Drawing for the job (mm, zero at the part's lowest x, y, z). A direction names the side the tool comes from. Round coordinates to 2 decimals unless told otherwise and drop trailing zeros. Order: outer loops, then holes, each group sorted by start corner. A loop starts at its lowest first (then second) coordinate and runs counter-clockwise, first axis right, second up. Notation, with made-up numbers: (85, 75) - (91, 75) arc R22 ccw to (91, 113) - close; hole circle Ø6 at (59.5, 44). An arc over 180 degrees is marked (long way). One line per question, with ' | ' between items. Start each with the question number.
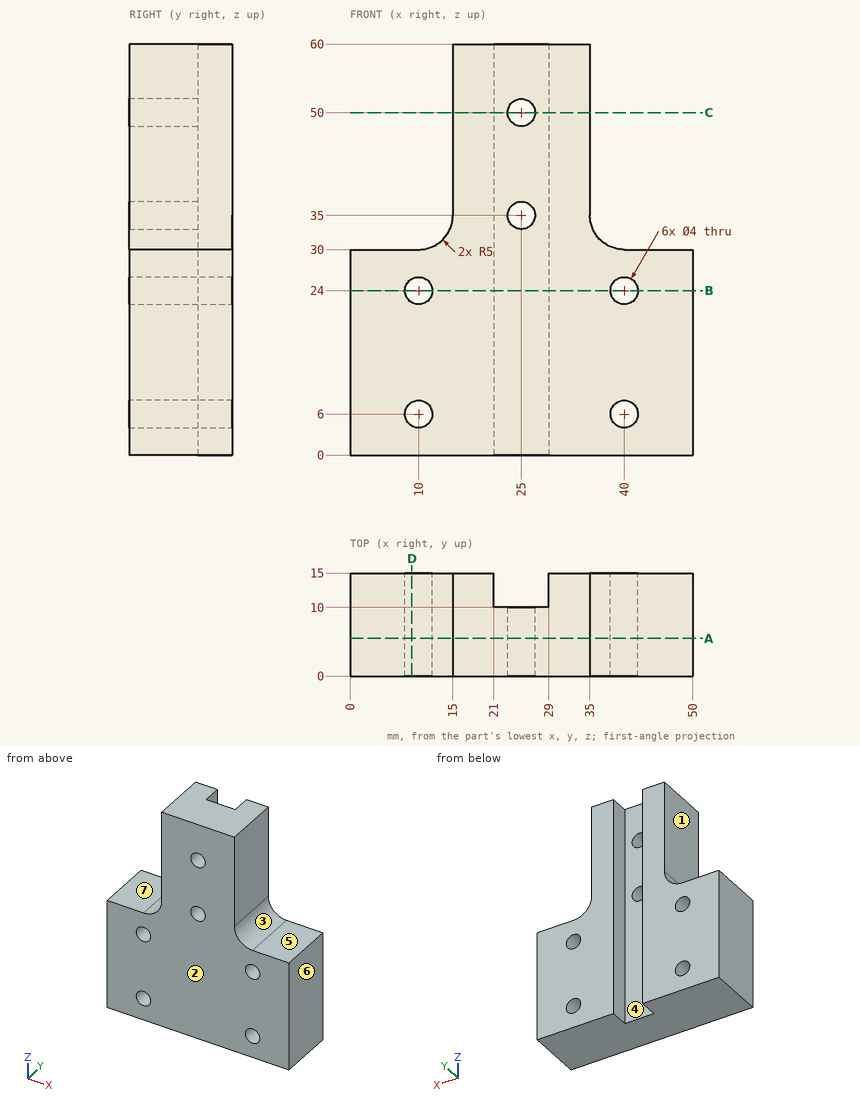
Item 1: Slice it at C-C (z = 50). Write the cut outline in (x, y).
Item 2: Wall check: line 1 along X through (y, z) = (5.75, 24); line 2 along X through (y, z) = (13, 37); line 3 along X through (y, z) = (2, 50). Give the ranges that are in metal, low to high. Write a range as [from, to].
Item 3: Pull direction X, two halves, no side cores. Call the marked faces 1, 2, 3 and 4: released by +X, released by -X, zero draft, split by the parting line, or undercut.
Item 4: 3-axis set-ups, long thin cutter, end or side, ignore diameter. For the marked faces 5, 6 and 7: which of +Z, -Z, +X, -X, +Y, -Y reach the whole face in a straight line?
Item 5: Pin check, flat tips, straight feed: pin 1 (7.5 mm diameter, centred on y = 9.5, z = 45, fed in from +X); pin 2 (5 mm diameter, centred on x = 25, z = 35, fed in from +Y); pin 3 (9 mm diameter, centred on x = 23.5, z = 21.5, fed in from +Y); pin 4 (8 mm diameter, centred on x = 47, y = 6.5, fed in from +Z). Stop position of each tip, or through.
Item 6: Slice it at D-D (x = 9). Write the cut outline in (y, z), plus the area to 3 significant figures.
Item 7: Slice it at B-B (z = 24). Write the cut outline in (x, y).
Item 8: Slice it at A-A (y = 5.5). Write the cut outline in (x, z), plus the area to 3 significant figures.
A:
1) outline: (15, 0) - (23, 0) - (23, 10) - (21, 10) - (21, 15) - (15, 15) - close; (27, 0) - (35, 0) - (35, 15) - (29, 15) - (29, 10) - (27, 10) - close
2) line 1: [0, 8], [12, 38], [42, 50] | line 2: [15, 21], [29, 35] | line 3: [15, 23], [27, 35]
3) face 1: released by -X | face 2: zero draft | face 3: released by +X | face 4: undercut
4) face 5: +Z, +X, +Y, -Y | face 6: +Z, -Z, +X, +Y, -Y | face 7: +Z, -X, +Y, -Y
5) pin 1: x = 35 | pin 2: y = 10 | pin 3: y = 15 | pin 4: z = 30
6) outline: (0, 0) - (15, 0) - (15, 4.27) - (0, 4.27) - close; (0, 7.73) - (15, 7.73) - (15, 22.27) - (0, 22.27) - close; (0, 25.73) - (15, 25.73) - (15, 30) - (0, 30) - close | area: 346 mm^2
7) outline: (0, 0) - (8, 0) - (8, 15) - (0, 15) - close; (12, 0) - (38, 0) - (38, 15) - (29, 15) - (29, 10) - (21, 10) - (21, 15) - (12, 15) - close; (42, 0) - (50, 0) - (50, 15) - (42, 15) - close
8) outline: (0, 0) - (50, 0) - (50, 30) - (40, 30) arc R5 cw to (35, 35) - (35, 60) - (15, 60) - (15, 35) arc R5 cw to (10, 30) - (0, 30) - close; hole circle Ø4 at (10, 6); hole circle Ø4 at (10, 24); hole circle Ø4 at (25, 35); hole circle Ø4 at (25, 50); hole circle Ø4 at (40, 6); hole circle Ø4 at (40, 24) | area: 2,040 mm^2
